```python
from build123d import *

# Parameters (mm, degrees)
EXTRUDE_1_DEPTH = 15
SCALE1_SCALE    = 2


with BuildPart() as part:
    # 草图1 → 凸台-拉伸1 (new, symmetric)
    with BuildSketch(Plane(origin=(0, 0, 0), x_dir=(1, 0, 0), z_dir=(0, 1, 0))):
        with BuildLine():
            Line((-39.222807174, 73.589999553), (103.277192826, 23.589999553))
            ThreePointArc((103.277192826, 23.589999553), (119.644979091, -4.198214571), (95, -25))
            Line((95, -25), (-95, -25))
            ThreePointArc((-95, -25), (-117.972466277, -9.862342174), (-113.12498584, 17.218736548))
            Line((-113.12498584, 17.218736548), (-65.62498584, 67.218736548))
            ThreePointArc((-65.62498584, 67.218736548), (-53.36455496, 74.302407188), (-39.222807174, 73.589999553))
        make_face()
        with BuildLine():
            Line((-61.999988672, 63.774989238), (-109.499988672, 13.774989238))
            ThreePointArc((-109.499988672, 13.774989238), (-113.377973022, -7.889873739), (-95, -20))
            Line((-95, -20), (95, -20))
            ThreePointArc((95, -20), (114.715983273, -3.358571657), (101.621754261, 18.871999643))
            Line((101.621754261, 18.871999643), (-40.878245739, 68.871999643))
            ThreePointArc((-40.878245739, 68.871999643), (-52.191643968, 69.44192575), (-61.999988672, 63.774989238))
        make_face(mode=Mode.SUBTRACT)
    extrude(amount=EXTRUDE_1_DEPTH, both=True)


with BuildPart() as part_1:
    # Scale1: scaled about (-2.797311239, 0, -12.318069734)
    add(part.part.scale(SCALE1_SCALE).moved(Location((2.797311239, 0, 12.318069734))))


solid = part_1.part
```
Here's how the part is built. I have some questions about the finished solid (model axes, mm). A direction names the side the tool comes from. Coordinates: 2 decimals unless noted, no trailing zeros. Order: outer loops, then holes, each group sorted by start corner. A loop starts at its lowest first (then second) coordinate and runs counter-clockwise, first axis right, second up. Notation, with made-up numbers: (-6, 65.25) -> (38, 65.25) arc R23 cw to (38, 79.25) -> close; hole circle Ø7 at (68, -36). An arc over 180 degrees is marked (long way). Return JSON: item names as keys, results as strings.
1) On a 3-axis mill with a long thin cutter (end or side, diameter ignored), from which of +Z, -Z, +X, -X, +Y, -Y can I reach the whole of each face in a straight line? I mean faces 4 (the cylindrical face through (232.09, 0.42, 19.81)), 5 (the cylindrical face through (242.24, 0.42, 19.75)). Say none if no direction works.
Conclusion:
{"face 4": "+Y, -Y", "face 5": "+X, +Y, -Y"}
2) I'm going to push flat-ended pins straight in: P1, Ø1, axis at y = -21, z = 12.5, coming from the -X side; P2, Ø18, axis at x = -38, y = -13, coming from the -Z side; P3, Ø12, axis at x = 149.5, z = -35, coming from the +Y side. Where does each tip first touch, or does it pass through?
Conclusion:
{"P1": "stops at x = -237.2", "P2": "stops at z = -124.81", "P3": "passes through"}
3) If we section it at C-C on z = 15: List the corners of the cut face in (x, y) for me.
Conclusion:
{"outline": "(-237.13, -30) -> (-227.11, -30) -> (-227.11, 30) -> (-237.13, 30) -> close; (232.71, -30) -> (242.73, -30) -> (242.73, 30) -> (232.71, 30) -> close"}
4) If we section it at A-A on y = -12: List the corners of the cut face in (x, z) for me.
Conclusion:
{"outline": "(-223.45, -22.12) -> (-128.45, -122.12) arc R50 ccw to (-75.65, -134.86) -> (209.35, -34.86) arc R50 ccw to (192.8, 62.32) -> (-187.2, 62.32) arc R50 ccw to start; hole (-216.2, -15.23) -> (-121.2, -115.23) arc R40 ccw to (-78.96, -125.43) -> (206.04, -25.43) arc R40 ccw to (192.8, 52.32) -> (-187.2, 52.32) arc R40 ccw to start"}
5) If I drill on probe 1 along Z at (x, y) = (-119, -16.5); probe 2 along Z at (x, y) = (1.5, -6.5); probe 3 along X at (y, z) = (4, 14), over which ranges is the centre line in solid material (lowest first)?
Conclusion:
{"probe 1": "z = -129.89 to -117.38, 52.32 to 62.32", "probe 2": "z = -107.79 to -97.19, 52.32 to 62.32", "probe 3": "x = -237.17 to -227.17, 232.76 to 242.77"}
6) Thinking about a two-plate mould opening in X: for faces 1 (the flat face through (4, 30, -97)), 2 (the flat face through (0, 0, 52.318)), 3 (the flat face through (-176.618, 0.42, -71.419)), which applies, +X half, -X half, draft (parallel to the pull), parting line (faces both ways), or undercut?
Conclusion:
{"face 1": "draft", "face 2": "undercut", "face 3": "-X half"}
7) If we section it at B-B on x = -191.5: List the corners of the cut face in (y, z) for me, plus the area to 3 significant figures.
Conclusion:
{"outline": "(-30, -55.75) -> (30, -55.75) -> (30, -41.23) -> (-30, -41.23) -> close; (-30, 52.09) -> (30, 52.09) -> (30, 62.13) -> (-30, 62.13) -> close", "area": "1,470 mm²"}
